Answer from the drawing. Dimensions are ordinates in mm from the lowest x, y and z of the part. A direction names the side the tool comes from. Round coordinates to 2 decimals unless told otherwise and drop trailing zeros. Loops run counter-clockwise (first coordinate to the right, second up) from the corner with the lowest first, then second, coordinate; pieces in that order, holes last. Notation, with made-up numbers: M -28.75,81.5 L 12.25,81.5 A21 cw 12.25,119.5 Z; hole C -34.75,-38.75 d5. An arc over 180 degrees is marked long. Write each question's results on one line, items separated by ' | '.
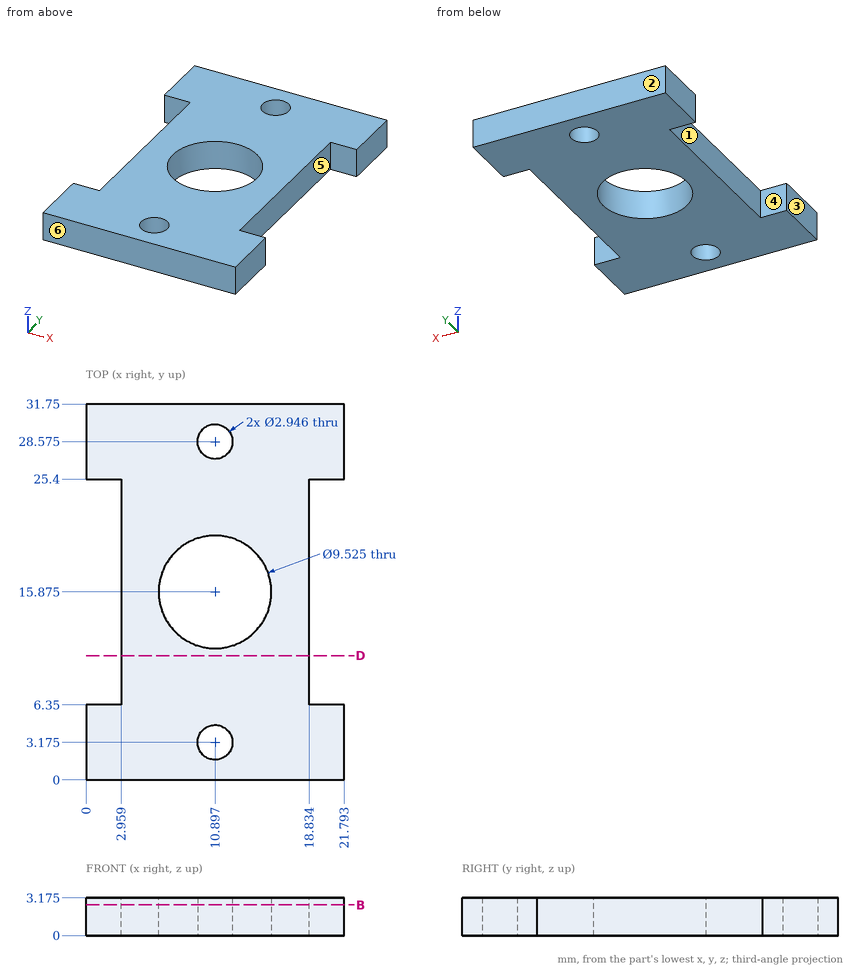
1. Which of the six approach directions +Z, -Z, +X, -X, +Y, -Y give full straight-line access (tool end or side, diameter ignored) to the marked faces 4, 5 and 6?
Completed:
face 4: +Z, -Z, -X | face 5: +Z, -Z, +X | face 6: +Z, -Z, +X, -X, -Y
2. Determine the mould class of the marked faces 1, 2 and 3 for opening direction Y: released by +Y, released by -Y, zero draft, split by the parting line, or undercut.
Completed:
face 1: undercut | face 2: released by +Y | face 3: zero draft
3. Given P1, Ø1.5, axis at x = 1.5, z = 2.5, coming from the -Y side; P2, Ø1, axis at y = 12, z = 1.5, coming from the +X side; P3, Ø2.5, axis at x = 10.9, y = 28.58, coming from the -Z side; P4, Ø1.6, axis at y = 15, z = 1, coming from the -X side, each flat-ended and moving along its own axis, determine where each tip first touches the part or whether it passes through.
Completed:
P1: stops at y = 0 | P2: stops at x = 18.83 | P3: passes through | P4: stops at x = 2.96
4. Find section D-D, the plane y = 10.5. Give the vertices of the cut face in (x, z) (1 decimal).
Completed:
outline: M 3,0 L 18.8,0 L 18.8,3.2 L 3,3.2 Z
5. Find section B-B, the plane z = 2.6. Count the separate pieces of the cut face and the enclosed holes in it, then the cut area to 3 significant figures.
Completed:
separate pieces: 1 | enclosed holes: 3 | area: 494 mm2
6. Find the intervals of material crossed by L1, parallel to Y at x = 20.5, z = 0.3; L2, parallel to X at y = 7, z = 1.5; L3, parallel to X at y = 28, z = 1, in increasing order.
Completed:
L1: y = 0 to 6.35, 25.4 to 31.75 | L2: x = 2.96 to 18.83 | L3: x = 0 to 9.54, 12.25 to 21.79
